Geometry check sheet. Reference: the model listing, model coordinates, mm. Face numbers are marked on the shaded views. A direction names the side the tool comes from. Round coordinates to 2 decimals unless told otherwise and drop trailing zeros. Write each loop counter-clockwise with the first axis right and the second up, starting at its lowest first coordinate (ties: lowest second). Pieces come first, ordered by that corner, then holes. Notation, with made-up numbers: (89.25, -27.5) -> (93.25, -27.5) arc R21 ccw to (93.25, -21.5) -> close; hole circle Ø4 at (7, 76.5). An arc over 180 degrees is marked (long way). One line per question, with ' | ' between items.
```python
from build123d import *

# Parameters (mm, degrees)
CUT_EXTRUDE1_DEPTH      = 41.7416
SKETCH3_R               = 1.5875
CUT_EXTRUDE2_DEPTH      = 17.51
CUT_EXTRUDE2_DEPTH_BACK = 17.51


with BuildPart() as part:
    # Sketch1 → Revolve1 (revolve)
    with BuildSketch(Plane.XY):
        Polygon((-7.62, 18.3642), (-16.51, 18.3642), (-16.51, 17.0942), (-12.7, 17.0942), (-12.7, -17.0942), (-16.51, -17.0942), (-16.51, -18.3642), (-7.62, -18.3642), (-7.62, -20.3708), (0, -20.3708), (0, 20.3708), (-7.62, 20.3708), align=None)
    revolve(axis=Axis((0, 20.3708, 0), (0, -1, 0)))

    # Sketch2 → Cut-Extrude1 (cut, through all)
    with BuildSketch(Plane(origin=(0, 20.3708, 0), x_dir=(1, 0, 0), z_dir=(0, 1, 0))):
        Polygon((0, 5.499261314), (-4.7625, 2.749630657), (-4.7625, -2.749630657), (0, -5.499261314), (4.7625, -2.749630657), (4.7625, 2.749630657), align=None)
    extrude(amount=-CUT_EXTRUDE1_DEPTH, mode=Mode.SUBTRACT)

    # Sketch3 → Cut-Extrude2 (cut, two sides)
    with BuildSketch(Plane(origin=(0, 0, 0), x_dir=(0, 0, -1), z_dir=(1, 0, 0))) as cut_extrude2_sk:
        with Locations((0, 12.7)):
            Circle(SKETCH3_R)
    extrude(amount=CUT_EXTRUDE2_DEPTH, mode=Mode.SUBTRACT)
    extrude(cut_extrude2_sk.sketch, amount=-CUT_EXTRUDE2_DEPTH_BACK, mode=Mode.SUBTRACT)


solid = part.part
```
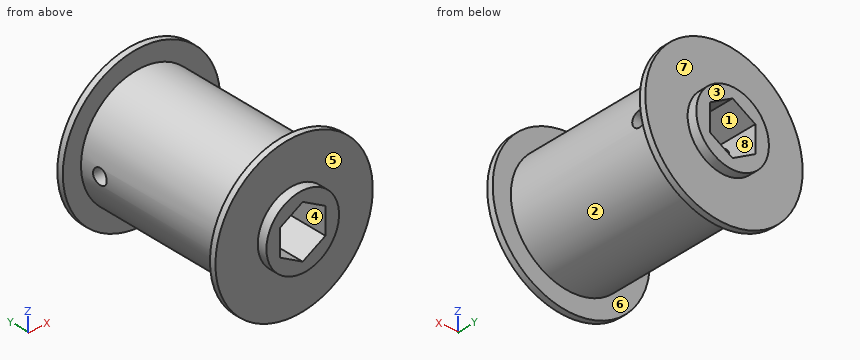
(1) Sectioned sample at C-C on x = -1.5. Record the cut outline in (y, z).
Resolved:
outline: (-20.37, -7.47) -> (-18.36, -7.47) -> (-18.36, -16.44) -> (-17.09, -16.44) -> (-17.09, -12.61) -> (17.09, -12.61) -> (17.09, -16.44) -> (18.36, -16.44) -> (18.36, -7.47) -> (20.37, -7.47) -> (20.37, -4.63) -> (-20.37, -4.63) -> close; (-20.37, 4.63) -> (20.37, 4.63) -> (20.37, 7.47) -> (18.36, 7.47) -> (18.36, 16.44) -> (17.09, 16.44) -> (17.09, 12.61) -> (-17.09, 12.61) -> (-17.09, 16.44) -> (-18.36, 16.44) -> (-18.36, 7.47) -> (-20.37, 7.47) -> close
(2) Sectioned sample at D-D on y = 12.7. Record the cut outline in (x, z), then the cut area to 3 significant figures.
Resolved:
outline: (-12.6, -1.59) arc R12.7 ccw to (12.6, -1.59) -> (4.76, -1.59) -> (4.76, -2.75) -> (0, -5.5) -> (-4.76, -2.75) -> (-4.76, -1.59) -> close; (-12.6, 1.59) -> (-4.76, 1.59) -> (-4.76, 2.75) -> (0, 5.5) -> (4.76, 2.75) -> (4.76, 1.59) -> (12.6, 1.59) arc R12.7 ccw to start | area: 378 mm2
(3) Sectioned sample at B-B on y = 4.5. Record the cut outline in (x, z).
Resolved:
outline: circle Ø25.4 at (0, 0); hole (-4.76, -2.75) -> (0, -5.5) -> (4.76, -2.75) -> (4.76, 2.75) -> (0, 5.5) -> (-4.76, 2.75) -> close
(4) Draft check along Z on the marked faces 1, 2, 3 and 4. Enter one of: +Z half, -Z half, draft (parallel to the pull), parting line (faces both ways), or undercut.
Resolved:
face 1: undercut | face 2: parting line | face 3: draft | face 4: undercut
(5) Go/stop test with flat-tipped pins: pin 1 (2.5 mm diameter, centred on y = -8, z = -0.5, fed in from +X); pin 2 (6 mm diameter, centred on x = 10, y = 7.5, fed in from +Z); pin 3 (5 mm diameter, centred on x = 2.5, y = -11.5, fed in from -Z). Record where each tip stops, or that it passes through.
Resolved:
pin 1: stops at x = 12.7 | pin 2: stops at z = 10.6 | pin 3: stops at z = -12.7
(6) Sectioned sample at A-A on z = 0. Count the separate pieces of the cut face and the enclosed holes in it, then the cut area to 3 significant figures.
Resolved:
separate pieces: 4 | enclosed holes: 0 | area: 575 mm2
(7) Material ranges on line 1 (Y direction, x = 9, z = 0); line 2 (Y direction, x = 2.5, z = 14.5); line 3 (Y direction, x = 6, z = -11), recorded low to high.
Resolved:
line 1: y = -18.36 to 11.11, 14.29 to 18.36 | line 2: y = -18.36 to -17.09, 17.09 to 18.36 | line 3: y = -18.36 to 18.36
(8) Access from +Z, -Z, +X, -X, +Y, -Y to the whole of each face (thin tool, end or side, straight path). Record for the marked faces 5, 6, 7 and 8.
Resolved:
face 5: -Y | face 6: none | face 7: +Y | face 8: +Y, -Y
